```python
from build123d import *

# Parameters (mm, degrees)
BOSS_EXTRUDE1_DEPTH                               = 1.5
BOSS_EXTRUDE2_DEPTH                               = 2.15
CSK_FOR_M2_5_FLAT_HEAD_MACHINE_SCREW1_D           = 2.8
CSK_FOR_M2_5_FLAT_HEAD_MACHINE_SCREW1_CSINK_D     = 5.5
CSK_FOR_M2_5_FLAT_HEAD_MACHINE_SCREW1_CSINK_ANGLE = 90
SKETCH6_R                                         = 6.05
CUT_EXTRUDE1_DEPTH                                = 4.65
SKETCH7_R                                         = 2.75
CUT_EXTRUDE2_DEPTH                                = 1
CSK_FOR_M2_5_FLAT_HEAD_MACHINE_SCREW2_D           = 2.9
CSK_FOR_M2_5_FLAT_HEAD_MACHINE_SCREW2_DEPTH       = 8
CSK_FOR_M2_5_FLAT_HEAD_MACHINE_SCREW2_CSINK_D     = 5.5
CSK_FOR_M2_5_FLAT_HEAD_MACHINE_SCREW2_CSINK_ANGLE = 90
CSK_FOR_M2_5_FLAT_HEAD_MACHINE_SCREW2_TIP         = 0.871247898


with BuildPart() as part:
    # Sketch1 → Boss-Extrude1 (new body)
    with BuildSketch(Plane(origin=(0, 0, 0), x_dir=(1, 0, 0), z_dir=(0, 1, 0))):
        with BuildLine():
            Line((-12.039826938, -3.360441535), (-6, -25))
            Line((-6, -25), (6, -25))
            Line((6, -25), (12.039826938, -3.360441535))
            ThreePointArc((12.039826938, -3.360441535), (0, 12.5), (-12.039826938, -3.360441535))
        make_face()
    extrude(amount=BOSS_EXTRUDE1_DEPTH)

    # Sketch2 → Boss-Extrude2 (add)
    with BuildSketch(Plane(origin=(0, 1.5, 0), x_dir=(1, 0, 0), z_dir=(0, 1, 0))):
        with BuildLine():
            Line((-6, -25), (-6, -12.093386622))
            ThreePointArc((-6, -12.093386622), (0, -13.5), (6, -12.093386622))
            Line((6, -12.093386622), (6, -25))
            Line((6, -25), (-6, -25))
        make_face()
    extrude(amount=BOSS_EXTRUDE2_DEPTH)

    # CSK for M2.5 Flat Head Machine Screw1 (through all)
    with Locations(Plane(origin=(0, 0, 0), x_dir=(-1, 0, 0), z_dir=(0, -1, 0))):
        with Locations((0, -9), (9, 0), (0, 9), (-9, 0)):
            CounterSinkHole(CSK_FOR_M2_5_FLAT_HEAD_MACHINE_SCREW1_D / 2, CSK_FOR_M2_5_FLAT_HEAD_MACHINE_SCREW1_CSINK_D / 2, counter_sink_angle=CSK_FOR_M2_5_FLAT_HEAD_MACHINE_SCREW1_CSINK_ANGLE)

    # Sketch6 → Cut-Extrude1 (cut, through all)
    with BuildSketch(Plane.XZ):
        Circle(SKETCH6_R)
    extrude(amount=-CUT_EXTRUDE1_DEPTH, mode=Mode.SUBTRACT)

    # Sketch7 → Cut-Extrude2 (cut)
    with BuildSketch(Plane(origin=(0, 0, 0), x_dir=(-1, 0, 0), z_dir=(0, -1, 0))):
        with Locations((0, -20)):
            Circle(SKETCH7_R)
    extrude(amount=-CUT_EXTRUDE2_DEPTH, mode=Mode.SUBTRACT)

    # CSK for M2.5 Flat Head Machine Screw2
    with Locations(Plane(origin=(0, 1, 0), x_dir=(-1, 0, 0), z_dir=(0, -1, 0))):
        with Locations((0, -20)):
            CounterSinkHole(CSK_FOR_M2_5_FLAT_HEAD_MACHINE_SCREW2_D / 2, CSK_FOR_M2_5_FLAT_HEAD_MACHINE_SCREW2_CSINK_D / 2, depth=CSK_FOR_M2_5_FLAT_HEAD_MACHINE_SCREW2_DEPTH, counter_sink_angle=CSK_FOR_M2_5_FLAT_HEAD_MACHINE_SCREW2_CSINK_ANGLE)
            with Locations((0, 0, -(CSK_FOR_M2_5_FLAT_HEAD_MACHINE_SCREW2_DEPTH + CSK_FOR_M2_5_FLAT_HEAD_MACHINE_SCREW2_TIP / 2))):  # 118° drill point
                Cone(0, CSK_FOR_M2_5_FLAT_HEAD_MACHINE_SCREW2_D / 2, CSK_FOR_M2_5_FLAT_HEAD_MACHINE_SCREW2_TIP, mode=Mode.SUBTRACT)


solid = part.part
```
For this review, take the finished solid that the model builds, in its own axes (mm). A direction names the side the tool comes from. Give positions to 0.01 mm unless a question says otherwise; leave off trailing zeros. Write each loop counter-clockwise with the first axis right and the second up, starting at its lowest first coordinate (ties: lowest second). Pieces come first, ordered by that corner, then holes. Notation, with made-up numbers: M 41,-22 L 86,-22 A25 ccw 86,9 Z; hole C 42,67 d5. An arc over 180 degrees is marked long. Answer as CSV lines item,"result".
1. For faces 1 (the flat face through (0, 3.65, 18)), 2 (the flat face through (-6, 3, 19)), 3 (the cylindrical face through (0.358, 0.493, 17.273)), list the 3-axis set-ups (+Z, -Z, +X, -X, +Y, -Y) from which the entire face can be reached by the end or side of a thin tool; tool diameter is ignored.
Findings:
face 1,"+Z, -Z, +X, -X, +Y"
face 2,"+Z, -Z, -X, +Y"
face 3,"-Y"
2. For pin 1 (8 mm diameter, centred on x = 8.5, z = 2.5, fed in from +Y); pin 2 (0.6 mm diameter, centred on y = 2.5, z = 21.5, fed in from +X); pin 3 (1.1 mm diameter, centred on y = 2.5, z = 21.5, fed in from -X), all flat-tipped, find the tip position at first contact; note any pin that passes through.
Findings:
pin 1,"stops at y = 1.5"
pin 2,"stops at x = 6"
pin 3,"stops at x = -6"
3. Consider section B-B, the plane y = 0.45. Write out the cut boundary in (x, z), then the cut area to 3 significant figures.
Findings:
outline,"M -12.04,3.36 A12.5 ccw long 12.04,3.36 L 6,25 L -6,25 Z; hole C -9,0 d4.6; hole C 0,0 d12.1; hole C 0,20 d5.5; hole C 0,-9 d4.6; hole C 0,9 d4.6; hole C 9,0 d4.6"
area,"514 mm2"
4. Consider section C-C, the plane z = 0. Write out the cut boundary in (x, y).
Findings:
outline,"M -12.5,0 L -11.75,0 L -10.4,1.35 L -10.4,1.5 L -12.5,1.5 Z; M -7.6,1.35 L -6.25,0 L -6.05,0 L -6.05,1.5 L -7.6,1.5 Z; M 6.05,0 L 6.25,0 L 7.6,1.35 L 7.6,1.5 L 6.05,1.5 Z; M 10.4,1.35 L 11.75,0 L 12.5,0 L 12.5,1.5 L 10.4,1.5 Z"
5. Consider section D-D, the plane x = 9. Write out the cut boundary in (y, z).
Findings:
outline,"M 0,-8.67 L 1.5,-8.67 L 1.5,-1.4 L 1.35,-1.4 L 0,-2.75 Z; M 0,2.75 L 1.35,1.4 L 1.5,1.4 L 1.5,14.25 L 0,14.25 Z"
6. Wall thickness on line 1 (Z direction, x = 0, y = 1.45); line 2 (Z direction, x = 0, y = 0.5); line 3 (Y direction, x = -9, z = -7): over which ranges is each line inside the solid? List them lowest first.
Findings:
line 1,"z = -12.5 to -10.4, -7.6 to -6.05, 6.05 to 7.6, 10.4 to 17.7, 22.3 to 25"
line 2,"z = -12.5 to -11.25, -6.75 to -6.05, 6.05 to 6.75, 11.25 to 17.25, 22.75 to 25"
line 3,"y = 0 to 1.5"
7. Consider section A-A, the plane x = 0. Count the separate pieces of the cut face and the enclosed holes in it, then the cut area to 3 significant figures.
Findings:
separate pieces,"5"
enclosed holes,"0"
area,"35.9 mm2"
8. Draft analysis for pull direction Z (two halves, no side actions). For faces 4 (the flat face through (-9.06, 0.74, 14.03)), 5 (the cylindrical face through (5.589, 0.74, -2.317)), 6 (the cylindrical face through (-0.314, 2.984, 21.416)), 7 (the flat face through (-3, 0, 6)), state which applies: +Z half, -Z half, draft (parallel to the pull), parting line (faces both ways), or undercut.
Findings:
face 4,"+Z half"
face 5,"undercut"
face 6,"undercut"
face 7,"draft"
